```python
from build123d import *

# Parameters (mm, degrees)
SKETCH1_R           = 3.75
BOSS_EXTRUDE1_DEPTH = 7
SKETCH2_R           = 3.75
SKETCH2_R_2         = 2.5
CUT_EXTRUDE1_DEPTH  = 4
SKETCH3_R           = 1.65
BOSS_EXTRUDE2_DEPTH = 2


with BuildPart() as part:
    # Sketch1 → Boss-Extrude1 (new body)
    with BuildSketch(Plane(origin=(0, 0, 0), x_dir=(1, 0, 0), z_dir=(0, 1, 0))):
        Circle(SKETCH1_R)
    extrude(amount=BOSS_EXTRUDE1_DEPTH)

    # Sketch2 → Cut-Extrude1 (cut)
    with BuildSketch(Plane(origin=(0, 7, 0), x_dir=(1, 0, 0), z_dir=(0, 1, 0))):
        Circle(SKETCH2_R)
        Circle(SKETCH2_R_2, mode=Mode.SUBTRACT)
    extrude(amount=-CUT_EXTRUDE1_DEPTH, mode=Mode.SUBTRACT)

    # Sketch3 → Boss-Extrude2 (add)
    with BuildSketch(Plane(origin=(0, 7, 0), x_dir=(1, 0, 0), z_dir=(0, 1, 0))):
        Circle(SKETCH3_R)
    extrude(amount=BOSS_EXTRUDE2_DEPTH)


solid = part.part
```
CAD build for the part. Positions are in the model's coordinates, mm. A direction names the side the tool comes from. Round coordinates to 2 decimals unless told otherwise and drop trailing zeros. Order: outer loops, then holes, each group sorted by start corner. A loop starts at its lowest first (then second) coordinate and runs counter-clockwise, first axis right, second up. Notation, with made-up numbers: (-5.5, -9.5) - (1.5, -9.5) arc R8 cw to (1.5, 5.5) - close; hole circle Ø9 at (40, 23.5). An arc over 180 degrees is marked (long way). Answer as CSV lines item,"result". Start each with the question number.
1. Saw through at C-C, the plane y = 5.75. Write the cut outline in (x, z), and give its area (3 significant figures).
2. Saw through at A-A, the plane x = 0. Write the cut outline in (y, z).
3. Drill centre lines: L1, parallel to Y at x = -1.25, z = -2.5; L2, parallel to Y at x = 2, z = -0.5; L3, parallel to X at y = 6.5, z = 0.5. Where is each one in solid material? Low to high. Write a range as [from, to].
4. Saw through at D-D, the plane x = -3. Write the cut outline in (y, z).
5. Pin check, flat tips, straight feed: pin 1 (1 mm diameter, centred on x = 0.5, y = 7, fed in from +Z); pin 2 (1 mm diameter, centred on y = 2.5, z = 1, fed in from +X). Stop position of each tip, or through.
6. Tool access for faces 1 (the face through (0, 9, 0)), 2 (the face through (-0.54, 5.03, 2.44)): list every direction of +Z, -Z, +X, -X, +Y, -Y with a clear straight run to the whole face (end or side of a thin tool).
7. Saw through at B-B, the plane z = 0. Write the cut outline in (x, y).
Model answer:
1,outline,"circle Ø5 at (0, 0)"
1,area,"19.6 mm²"
2,outline,"(0, -3.75) - (3, -3.75) - (3, -2.5) - (7, -2.5) - (7, -1.65) - (9, -1.65) - (9, 1.65) - (7, 1.65) - (7, 2.5) - (3, 2.5) - (3, 3.75) - (0, 3.75) - close"
3,L1,"y = [0, 3]"
3,L2,"y = [0, 7]"
3,L3,"x = [-2.45, 2.45]"
4,outline,"(0, -2.25) - (3, -2.25) - (3, 2.25) - (0, 2.25) - close"
5,pin 1,"stops at z = 2.5"
5,pin 2,"stops at x = 3.72"
6,face 1,"+Z, -Z, +X, -X, +Y"
6,face 2,"+Y"
7,outline,"(-3.75, 0) - (3.75, 0) - (3.75, 3) - (2.5, 3) - (2.5, 7) - (1.65, 7) - (1.65, 9) - (-1.65, 9) - (-1.65, 7) - (-2.5, 7) - (-2.5, 3) - (-3.75, 3) - close"
